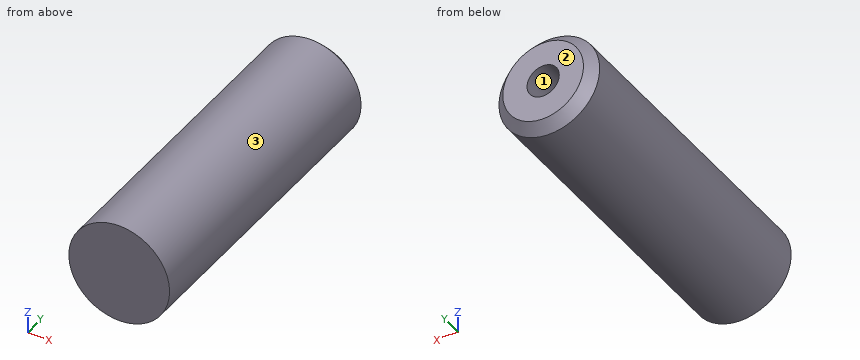
```python
from build123d import *

# Parameters (mm, degrees)
ESQUISSE1_R             = 2.5
BOSS_EXTRU_1_DEPTH      = 6
BOSS_EXTRU_1_DEPTH_BACK = 10
TROU_TARAUD_M21_D       = 1.6
TROU_TARAUD_M21_DEPTH   = 6
TROU_TARAUD_M21_TIP     = 0.480688495
CHANFREIN1_SIZE         = 0.5


with BuildPart() as part:
    # Esquisse1 → Boss.-Extru.1 (new body, two sides)
    with BuildSketch(Plane(origin=(0, 0, 0), x_dir=(1, 0, 0), z_dir=(0, 1, 0))) as boss_extru_1_sk:
        Circle(ESQUISSE1_R)
    extrude(amount=BOSS_EXTRU_1_DEPTH)
    extrude(boss_extru_1_sk.sketch, amount=-BOSS_EXTRU_1_DEPTH_BACK)

    # Trou taraudé M21
    with Locations(Plane(origin=(0, 6, 0), x_dir=(1, 0, 0), z_dir=(0, 1, 0))):
        with Locations((0, 0)):
            Hole(TROU_TARAUD_M21_D / 2, depth=TROU_TARAUD_M21_DEPTH)
            with Locations((0, 0, -(TROU_TARAUD_M21_DEPTH + TROU_TARAUD_M21_TIP / 2))):  # 118° drill point
                Cone(0, TROU_TARAUD_M21_D / 2, TROU_TARAUD_M21_TIP, mode=Mode.SUBTRACT)

    # Chanfrein1
    chanfrein1_edges = [part.edges().sort_by_distance(p)[0] for p in [
        (-2.5, 6, 0),
    ]]
    chamfer(chanfrein1_edges, length=CHANFREIN1_SIZE)


solid = part.part
```
Source: CAD feature listing. Evaluate the final solid. Frame: model axes, mm. Face numbers are marked on the shaded views. Round coordinates to 2 decimals unless told otherwise and drop trailing zeros. Write each loop counter-clockwise with the first axis right and the second up, starting at its lowest first coordinate (ties: lowest second). Pieces come first, ordered by that corner, then holes. Notation, with made-up numbers: M 60.5,-14 L 78.5,-14 A35 cw 78.5,25 Z; hole C -29,37 d6. An arc over 180 degrees is marked long. Answer as a JSON object with one key per item and string values. Group by question number.
(1) Mould query, pull axis Z, two halves, no side actions, for the marked faces 1, 2 and 3. Classes: +Z half, -Z half, draft (parallel to the pull), parting line (faces both ways), or undercut.
(2) Section query A-A on y = 4.25. Output: boundary loops of the cut face in (x, z), then the cut area to 3 significant figures.
(3) Section query B-B on y = -8.75. Output: boundary loops of the cut face in (x, z), then the cut area to 3 significant figures.
(4) Ray query, line 1 (Z direction, x = 0, y = 3.3); line 2 (Z direction, x = 0.6, y = 3.5); line 3 (Y direction, x = -1.8, z = -1.3). Return the intervals inside material, ascending. Write a range as [from, to].
(5) First-contact query: pin 1 (2 mm diameter, centred on y = -3, z = 1.5, fed in from -X); pin 2 (2 mm diameter, centred on x = 1.5, y = 3.5, fed in from -Z). Flat tips, straight axial feed; report the tip coordinate or a pass-through.
Computed values:
{
 "1": {"face 1": "undercut", "face 2": "draft", "face 3": "parting line"},
 "2": {"outline": "C 0,0 d5; hole C 0,0 d1.6", "area": "17.6 mm^2"},
 "3": {"outline": "C 0,0 d5", "area": "19.6 mm^2"},
 "4": {"line 1": "[-2.5, -0.8], [0.8, 2.5]", "line 2": "[-2.43, -0.53], [0.53, 2.43]", "line 3": "[-10, 5.78]"},
 "5": {"pin 1": "x = -2.45", "pin 2": "z = -2.45"}
}
